Design review of the part built by this model. Coordinates are the model's own, in mm. A direction names the side the tool comes from. Give positions to 0.01 mm unless a question says otherwise; leave off trailing zeros. Loops run counter-clockwise (first coordinate to the right, second up) from the corner with the lowest first, then second, coordinate; pieces in that order, holes last. Notation, with made-up numbers: (-27, 77.25) -> (16, 77.25) arc R32 cw to (16, 110.25) -> close; hole circle Ø10 at (87.25, -10). An arc over 180 degrees is marked (long way). Answer in a Markdown table with one row per item. Add a question column.
(1) Consider section C-C on z = 23. Write out the cut boundary in (x, y) (3 decimals).
(2) For pin 1 (3 mm diameter, centred on x = 0, z = 3.5, fed in from +Y); pin 2 (5 mm diameter, centred on x = -17, z = 3, fed in from +Y); pin 3 (3 mm diameter, centred on x = 1, z = 25.5, fed in from -Y) (3 decimals); pin 4 (1.5 mm diameter, centred on y = 0.5, z = 16, fed in from +X) (3 decimals), all flat-tipped, find the tip position at first contact; note any pin that passes through.
(3) Consider section D-D on y = -3. Write out the cut boundary in (x, z).
(4) Consider section A-A on z = 3.5. Write out the cut boundary in (x, y).
(5) Draft analysis for pull direction Z (two halves, no side actions). For faces 6 (the cylindrical face through (-0.27, 10, 2.28)), 7 (the flat face through (5.3, 0.2, 37)), 8 (the flat face through (-16, -5.13, 3)), 9 (the cylindrical face through (-0.202, -9.997, 1.963)), state which applies: +Z half, -Z half, draft (parallel to the pull), parting line (faces both ways), or undercut.
(6) Consider section B-B on x = 0. Write out the cut boundary in (y, z) (3 decimals).
(7) For faces 1 (the flat face through (0, 5.13, 18)), 2 (the flat face through (-16, 5.13, 3)), 3 (the flat face through (-13, -1, 7)), 4 (the flat face through (-9, 0, 0)), 5 (the cylindrical face through (-22.156, -3.626, 3.549)), list the 3-axis set-ups (+Z, -Z, +X, -X, +Y, -Y) from which the entire face can be reached by the end or side of a thin tool; tool diameter is ignored.
(8) For line 1 (Z direction, x = 0, y = 8.25); line 2 (Z direction, x = 0, y = -9.25); line 3 (Y direction, x = 0, z = 14) (3 decimals), list the stretches that pass through material, from the lowest coordinate up.
from build123d import *

# Parameters (mm, degrees)
F1_DEPTH = 7
F2_DEPTH = 37
F4_D     = 2.5
F4_DEPTH = 9.871
F5_D     = 3.1
F5_DEPTH = 20.1310001
F6_R     = 5
F7_D     = 2.5


with BuildPart() as f1:
    # F0 (on Top) → F1 (new body)
    with BuildSketch(Plane.XY):
        with BuildLine():
            ThreePointArc((-14.0954992817, -5.13), (2.6045643373, -14.7721442117), (15, 0))
            ThreePointArc((15, 0), (2.6045643373, 14.7721442117), (-14.0954992817, 5.13))
            Line((-14.0954992817, 5.13), (-11.2725917605, 5.13))
            ThreePointArc((-11.2725917605, 5.13), (2.6246119757, 12.1037034406), (12.385, 0))
            ThreePointArc((12.385, 0), (2.6246119757, -12.1037034406), (-11.2725917605, -5.13))
            Line((-11.2725917605, -5.13), (-14.0954992817, -5.13))
        make_face()
        with BuildLine():
            Line((-11.2725917605, 5.13), (-14.0954992817, 5.13))
            ThreePointArc((-14.0954992817, 5.13), (-15, 0), (-14.0954992817, -5.13))
            Line((-14.0954992817, -5.13), (-11.2725917605, -5.13))
            ThreePointArc((-11.2725917605, -5.13), (-12.385, 0), (-11.2725917605, 5.13))
        make_face()
        with BuildLine():
            ThreePointArc((12.385, 0), (2.6246119757, 12.1037034406), (-11.2725917605, 5.13))
            Line((-11.2725917605, 5.13), (-5.13, 5.13))
            Line((-5.13, 5.13), (5.13, 5.13))
            Line((5.13, 5.13), (5.13, -5.13))
            Line((5.13, -5.13), (-5.13, -5.13))
            Line((-5.13, -5.13), (-11.2725917605, -5.13))
            ThreePointArc((-11.2725917605, -5.13), (2.6246119757, -12.1037034406), (12.385, 0))
        make_face()
        with BuildLine():
            Line((-5.13, 5.13), (-11.2725917605, 5.13))
            ThreePointArc((-11.2725917605, 5.13), (-12.385, 0), (-11.2725917605, -5.13))
            Line((-11.2725917605, -5.13), (-5.13, -5.13))
            Line((-5.13, -5.13), (-5.13, 5.13))
        make_face()
        with BuildLine():
            ThreePointArc((-14.0954992817, -5.13), (-15, 0), (-14.0954992817, 5.13))
            Line((-14.0954992817, 5.13), (-23.5814342785, 5.13))
            Line((-23.5814342785, 5.13), (-23.5814342785, 0))
            Line((-23.5814342785, 0), (-23.5814342785, -5.13))
            Line((-23.5814342785, -5.13), (-14.0954992817, -5.13))
        make_face()
    extrude(amount=F1_DEPTH)

    # F0 (on Top) → F2 (join)
    with BuildSketch(Plane.XY):
        with BuildLine():
            Line((-5.13, 5.13), (-11.2725917605, 5.13))
            ThreePointArc((-11.2725917605, 5.13), (-12.385, 0), (-11.2725917605, -5.13))
            Line((-11.2725917605, -5.13), (-5.13, -5.13))
            Line((-5.13, -5.13), (-5.13, 5.13))
        make_face()
        with BuildLine():
            ThreePointArc((12.385, 0), (2.6246119757, 12.1037034406), (-11.2725917605, 5.13))
            Line((-11.2725917605, 5.13), (-5.13, 5.13))
            Line((-5.13, 5.13), (5.13, 5.13))
            Line((5.13, 5.13), (5.13, -5.13))
            Line((5.13, -5.13), (-5.13, -5.13))
            Line((-5.13, -5.13), (-11.2725917605, -5.13))
            ThreePointArc((-11.2725917605, -5.13), (2.6246119757, -12.1037034406), (12.385, 0))
        make_face()
    extrude(amount=F2_DEPTH)

    # F4 (through all, one way)
    with BuildSketch(Plane.XZ.offset(-5.13)):
        with Locations((0, 3.5)):
            Circle(F4_D / 2)
    extrude(amount=-F4_DEPTH, mode=Mode.SUBTRACT)

    # F5 (through all, one way)
    with BuildSketch(Plane(origin=(0, 5.13, 0), x_dir=(1, 0, 0), z_dir=(0, 1, 0))):
        with Locations((0, -3.5)):
            Circle(F5_D / 2)
    extrude(amount=-F5_DEPTH, mode=Mode.SUBTRACT)

    # F6
    f6_edges = [f1.edges().sort_by_distance(p)[0] for p in [
        (-23.581434, -5.13, 3.5),
        (-23.581434, 5.13, 3.5),
    ]]
    fillet(f6_edges, radius=F6_R)

    # F7 (through all)
    with Locations(Plane(origin=(0, 0, 0), x_dir=(1, 0, 0), z_dir=(0, 0, -1))):
        with Locations((-20.0814342785, 0)):
            Hole(F7_D / 2)


solid = f1.part
Values follow:
| question | item | result |
|---|---|---|
| 1 | outline | circle Ø24.77 at (0, 0); hole (-5.13, -5.13) -> (5.13, -5.13) -> (5.13, 5.13) -> (-5.13, 5.13) -> close |
| 2 | pin 1 | y = 15 |
| 2 | pin 2 | y = 5.13 |
| 2 | pin 3 | y = -12.385 |
| 2 | pin 4 | x = 12.385 |
| 3 | outline | (-22.68, 0) -> (-5.13, 0) -> (-5.13, 37) -> (-12.02, 37) -> (-12.02, 7) -> (-22.68, 7) -> close; (5.13, 0) -> (14.7, 0) -> (14.7, 7) -> (12.02, 7) -> (12.02, 37) -> (5.13, 37) -> close |
| 4 | outline | (-23.58, -0.13) arc R5 ccw to (-18.58, -5.13) -> (-14.1, -5.13) arc R15 ccw to (-1.55, -14.92) -> (-1.55, -5.13) -> (-5.13, -5.13) -> (-5.13, 5.13) -> (-1.25, 5.13) -> (-1.25, 14.95) arc R15 ccw to (-14.1, 5.13) -> (-18.58, 5.13) arc R5 ccw to (-23.58, 0.13) -> close; (1.25, 5.13) -> (5.13, 5.13) -> (5.13, -5.13) -> (1.55, -5.13) -> (1.55, -14.92) arc R15 ccw to (1.25, 14.95) -> close; hole circle Ø2.5 at (-20.08, 0) |
| 5 | face 6 | undercut |
| 5 | face 7 | +Z half |
| 5 | face 8 | draft |
| 5 | face 9 | undercut |
| 6 | outline | (-15, 0) -> (-5.13, 0) -> (-5.13, 1.95) -> (-15, 1.95) -> close; (-15, 5.05) -> (-5.13, 5.05) -> (-5.13, 37) -> (-12.385, 37) -> (-12.385, 7) -> (-15, 7) -> close; (5.13, 0) -> (15, 0) -> (15, 2.25) -> (5.13, 2.25) -> close; (5.13, 4.75) -> (15, 4.75) -> (15, 7) -> (12.385, 7) -> (12.385, 37) -> (5.13, 37) -> close |
| 7 | face 1 | +Z, -Z |
| 7 | face 2 | +Z, -Z, -X, +Y |
| 7 | face 3 | +Z |
| 7 | face 4 | -Z, +X, -X, +Y, -Y |
| 7 | face 5 | +Z, -Z, -X, -Y |
| 8 | line 1 | 0 to 2.25, 4.75 to 37 |
| 8 | line 2 | 0 to 1.95, 5.05 to 37 |
| 8 | line 3 | -12.385 to -5.13, 5.13 to 12.385 |
